Design review of the part built by this model. Coordinates are the model's own, in mm. Face numbers are marked on the shaded views. A direction names the side the tool comes from. Coordinates: 2 decimals unless noted, no trailing zeros. Write each loop counter-clockwise with the first axis right and the second up, starting at its lowest first coordinate (ties: lowest second). Pieces come first, ordered by that corner, then holes.
Q1. For probe 1 along X at (y, z) = (0.45, -0.6); probe 2 along Y at (x, z) = (2.5, 0.3); probe 3 along Y at (x, z) = (5.5, -0.4), list the stretches that pass through material, from the lowest coordinate up.
Q2. Take a section at A-A (x = 6.25). Give the boundary of the cut face in (y, z).
Q3. Machinability: for the marked faces 1 and 2, which of the approach directions +Z, -Z, +X, -X, +Y, -Y give a long, thin tool a straight path to every point of the face, cutting with its end or side? Answer none if there is none.
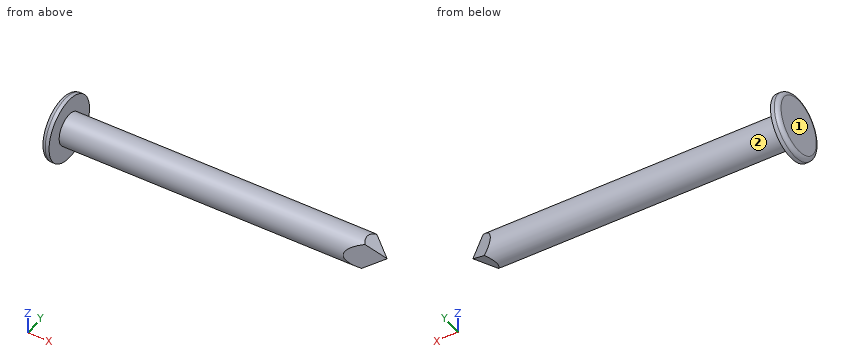
```python
from build123d import *

# Parameters (mm, degrees)
F0_R          = 0.5
F1_DEPTH      = 10
F0_R_2        = 1
F2_DEPTH      = 0.25
F3_R          = 0.13
F5_DEPTH      = 25
F5_DEPTH_BACK = 25
F7_DEPTH      = 25
F7_DEPTH_BACK = 25


with BuildPart() as f1:
    # F0 (on Right) → F1 (new body)
    with BuildSketch(Plane.YZ):
        Circle(F0_R)
    extrude(amount=F1_DEPTH)

    # F0 (on Right) → F2 (join)
    with BuildSketch(Plane.YZ):
        Circle(F0_R_2)
        Circle(F0_R, mode=Mode.SUBTRACT)
        Circle(F0_R)
    extrude(amount=-F2_DEPTH)

    # F3
    f3_edges = [f1.edges().sort_by_distance(p)[0] for p in [
        (-0.25, -1, 0),
    ]]
    fillet(f3_edges, radius=F3_R)

    # F4 (on Front) → F5 (cut, two sides)
    with BuildSketch(Plane.XZ) as f5_sk:
        Polygon((9.2973364517, 1.1940489057), (9.0074734762, 0.7828483358), (9.9916588515, 0), (8.8052442297, -0.7810618845), (10.7196858153, -0.7540978841), (10.7331676409, 1.3423507335), align=None)
    extrude(amount=-F5_DEPTH, mode=Mode.SUBTRACT)
    extrude(f5_sk.sketch, amount=F5_DEPTH_BACK, mode=Mode.SUBTRACT)

    # F6 (on Top) → F7 (cut, two sides)
    with BuildSketch(Plane.XY) as f7_sk:
        Polygon((9.9852262065, 0), (8.3366055042, -0.7803390617), (11.1771607772, -1.2145728106), (11.2198108528, 0.6940264138), (8.7891332805, 0.6940264138), align=None)
    extrude(amount=F7_DEPTH, mode=Mode.SUBTRACT)
    extrude(f7_sk.sketch, amount=-F7_DEPTH_BACK, mode=Mode.SUBTRACT)


solid = f1.part
```
Response:
1. probe 1: x = -0.25 to 0
1. probe 2: y = -0.4 to 0.4
1. probe 3: y = -0.3 to 0.3
2. outline: circle Ø1 at (0, 0)
3. face 1: +Z, -Z, -X, +Y, -Y
3. face 2: +X
